Work out the finished part from the listing and answer in its coordinate system (mm). Face numbers are marked on the shaded views. A direction names the side the tool comes from. Coordinates: 2 decimals unless noted, no trailing zeros. Order: outer loops, then holes, each group sorted by start corner. A loop starts at its lowest first (then second) coordinate and runs counter-clockwise, first axis right, second up. Notation, with made-up numbers: M 58.25,77 L 99.25,77 A15 cw 99.25,84 Z; hole C 52.25,0 d6. An arc over 180 degrees is marked long. Write item = value, one per line. Start each with the question number.
Q1. Straight lines are drawn through the part: line 1 along Y through (x, z) = (-16, 1.05); line 2 along X through (y, z) = (7, 2); line 3 along Z through (x, y) = (13, 24.5). For each, find the intervals that lie inside material, in ascending order.
Q2. A tool of negligible diameter and unlimited length cuts with its end or side. For the marked faces 1, 2, 3, 4 and 5, from which of +Z, -Z, +X, -X, +Y, -Y can it reach the whole face along a straight path? Write none if from no direction.
Q3. Find section B-B on x = -16. Give the vertices of the cut face in (y, z), and give its area (3 significant figures).
Q4. Find section D-D on y = 32.5. Give the vertices of the cut face in (x, z), and give its area (3 significant figures).
Q5. Find section A-A on y = 43.5. Give the vertices of the cut face in (x, z), and give its area (3 significant figures).
Q6. Each of these flat-tipped pins is pushed along its axis until it touches: P1, Ø24, axis at y = 32.5, z = 38, coming from the +X side; P2, Ø2, axis at y = 65, z = 28.5, coming from the -X side; P3, Ø6, axis at x = -8.5, y = 48, coming from the +Z side; P4, Ø6.5, axis at x = 16, y = 43.5, coming from the +Z side. Where does it stop, or does it pass through?
Q7. Find section C-C on z = 13.5. Give the vertices of the cut face in (x, y), and give its area (3 significant figures).
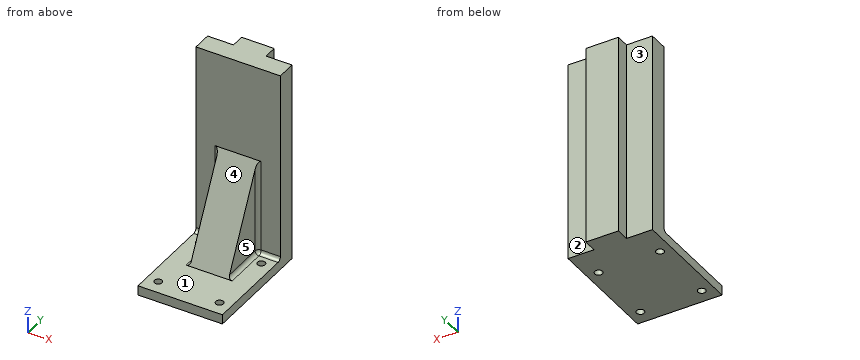
```python
from build123d import *

# Parameters (mm, degrees)
BOSS_EXTRUDE1_DEPTH = 5
SKETCH2_R           = 2
CUT_EXTRUDE1_DEPTH  = 5
SKETCH3_W           = 44
SKETCH3_H           = 10
BOSS_EXTRUDE2_DEPTH = 100
BOSS_EXTRUDE3_DEPTH = 10
FILLET1_R           = 2
SKETCH5_W           = 17
SKETCH5_H           = 105
BOSS_EXTRUDE4_DEPTH = 7


with BuildPart() as part:
    # Sketch1 → Boss-Extrude1 (new body)
    with BuildSketch(Plane.XY):
        Polygon((0, 0), (-22, 0), (-22, 60), (22, 60), (22, 0), align=None)
    extrude(amount=BOSS_EXTRUDE1_DEPTH)

    # Sketch2 → Cut-Extrude1 (cut)
    with BuildSketch(Plane(origin=(0, 0, 0), x_dir=(-1, 0, 0), z_dir=(0, 0, -1))):
        with Locations((-16, 43.5)):
            Circle(SKETCH2_R)
        with Locations((16, 43.5)):
            Circle(SKETCH2_R)
        with Locations((-16, 7.5)):
            Circle(SKETCH2_R)
        with Locations((16, 7.5)):
            Circle(SKETCH2_R)
    extrude(amount=-CUT_EXTRUDE1_DEPTH, mode=Mode.SUBTRACT)

    # Sketch3 → Boss-Extrude2 (add)
    with BuildSketch(Plane.XY.offset(5)):
        with Locations((0, 55)):
            Rectangle(SKETCH3_W, SKETCH3_H)
    extrude(amount=BOSS_EXTRUDE2_DEPTH)

    # Sketch4 → Boss-Extrude3 (add, symmetric)
    with BuildSketch(Plane(origin=(0, 0, 0), x_dir=(0, 0, -1), z_dir=(1, 0, 0))):
        Polygon((-5, 50), (-5, 25), (-55, 50), align=None)
    extrude(amount=BOSS_EXTRUDE3_DEPTH, both=True)

    # Fillet1
    fillet1_edges = [part.edges().sort_by_distance(p)[0] for p in [
        (16, 50, 5),
        (10, 37.5, 5),
        (10, 50, 30),
        (-16, 50, 5),
        (-10, 37.5, 5),
        (-10, 50, 30),
    ]]
    fillet(fillet1_edges, radius=FILLET1_R)

    # Sketch5 → Boss-Extrude4 (add)
    with BuildSketch(Plane(origin=(0, 60, 0), x_dir=(1, 0, 0), z_dir=(0, 1, 0))):
        with Locations((0, -52.5)):
            Rectangle(SKETCH5_W, SKETCH5_H)
    extrude(amount=BOSS_EXTRUDE4_DEPTH)


solid = part.part
```
Findings below:
q1.line_1 = 0 to 5.5, 9.5 to 41.5, 45.5 to 60
q1.line_2 = -22 to -17.94, -14.06 to 14.06, 17.94 to 22
q1.line_3 = 0 to 5
q2.face_1 = +Z, -Y
q2.face_2 = +Z, -Z, +X, +Y
q2.face_3 = +Z, -Z, -X, +Y
q2.face_4 = +Z, +X, -X, -Y
q2.face_5 = +Z, +X, -Y
q3.outline = M 0,0 L 5.5,0 L 5.5,5 L 0,5 Z; M 9.5,0 L 41.5,0 L 41.5,5 L 9.5,5 Z; M 45.5,0 L 60,0 L 60,105 L 50,105 L 50,7 A2 cw 48,5 L 45.5,5 Z
q3.area = 1,260 mm^2
q4.outline = M -22,0 L 22,0 L 22,5 L 12,5 A2 cw 10,7 L 10,20 L -10,20 L -10,7 A2 cw -12,5 L -22,5 Z
q4.area = 522 mm^2
q5.outline = M -22,0 L -18,0 L -18,5 L -22,5 Z; M -14,0 L 14,0 L 14,5 L 12,5 A2 cw 10,7 L 10,42 L -10,42 L -10,7 A2 cw -12,5 L -14,5 Z; M 18,0 L 22,0 L 22,5 L 18,5 Z
q5.area = 922 mm^2
q6.P1 = 10
q6.P2 = -8.5
q6.P3 = 105
q6.P4 = 5
q7.outline = M -22,50 L -12,50 A2 cw -10,48 L -10,29.25 L 10,29.25 L 10,48 A2 cw 12,50 L 22,50 L 22,60 L 8.5,60 L 8.5,67 L -8.5,67 L -8.5,60 L -22,60 Z
q7.area = 976 mm^2
